Geometry: final body of the model. Coordinates: model frame, mm. Round coordinates to 2 decimals unless told otherwise and drop trailing zeros. Write each loop counter-clockwise with the first axis right and the second up, starting at its lowest first coordinate (ties: lowest second). Pieces come first, ordered by that corner, then holes. Notation, with made-up numbers: M -40,38.5 L -32,38.5 A34 ccw -32,71.5 Z; hole C 13.25,56.5 d2. An arc over 180 degrees is marked long. Use one line per item in the form item = value. Start each with the question number.
Item 1: Section query C-C (y = 14.5). Return loops of the section in (x, z).
Item 2: Ray query, probe 1 along Y at (x, z) = (-27.5, 87); probe 2 along Y at (x, z) = (-12.5, 103). Return the intervals inside material, ascending.
Item 3: Section query A-A (x = -35.5). Return loops of the section in (y, z), and give its area (3 significant figures).
Item 4: Pin query (flat end, axial travel): pin 1 Ø8 at (x, z) = (-40, 92.5) entering from +Y; pin 2 Ø12 at (x, z) = (-35, 96) entering from +Y; pin 3 Ø2 at (x, z) = (-17, 94) entering from +Y. Return the tip coordinate at first contact, or that it passes through.
Item 5: Section query B-B (z = 98.5). Return loops of the section in (x, y), and give its area (3 significant figures).
Autodesk Inventor part; units mm, degrees
ref_plane "YZ Plane" through (0, 0, 0) normal (1, 0, 0) x (0, 1, 0)
ref_plane "XZ Plane" through (0, 0, 0) normal (0, 1, 0) x (-1, 0, 0)
ref_plane "XY Plane" through (0, 0, 0) normal (0, 0, 1) x (1, 0, 0)
sketch "Sketch1" plane through (0, 0, 0) normal (0, 0, 1) x (1, 0, 0)
  line L0 (38.1, 0) -> (-9.6364, 17.3746)
  line L1 (-9.6364, 17.3746) -> (-9.6364, 0)
  line L2 (-9.6364, 0) -> (38.1, 0)
  point P0 (0, 0)
  dimension "d2" = 50.8
  dimension "d4" = 70
extrude "Extrusion1" add sketch "Sketch1" along normal blind 38.1
move or copy body "Move Body1" bodies to move or copy 1 copy no rotation origin (0, 0, 0) rotation axis (0, 1, 0) rotation angle -180 translate (-19.2728, 0, 76.2)
move or copy body "Move Body2" bodies to move or copy 1 copy no rotation origin (0, 0, 0) rotation axis (0, 1, 0) rotation angle 90 translate (-85.8364, 0, 66.5636)
properties part number "70DegreeWoodHinge" material "Wood (Birch)"
Working result:
q1.outline = M -47.74,76.2 L -9.64,76.2 L -9.64,84.1 L -47.74,84.1 Z
q2.probe_1 = 0 to 13.44
q2.probe_2 = 0 to 7.62
q3.outline = M 0,76.2 L 17.37,76.2 L 0,123.94 Z
q3.area = 415 mm²
q4.pin_1 = 12.9
q4.pin_2 = 12.35
q4.pin_3 = 11.26
q5.outline = M -47.74,0 L -9.64,0 L -9.64,9.26 L -47.74,9.26 Z
q5.area = 353 mm²
